Read the model definition and answer for the solid it produces. Units are mm, in the model's axes. Coordinates: 2 decimals unless noted, no trailing zeros. Order: outer loops, then holes, each group sorted by start corner. A loop starts at its lowest first (then second) coordinate and runs counter-clockwise, first axis right, second up. Notation, with made-up numbers: (28.5, -21) - (68.5, -21) arc R13 ccw to (68.5, -4) - close; hole circle Ø11 at (-3.75, 26.5). An arc over 180 degrees is marked (long way). Answer as a JSON object with one key per item and string values. Group by question number.
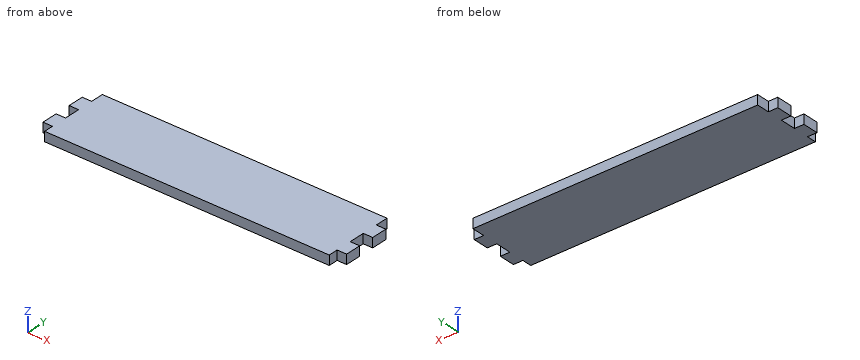
Autodesk Inventor part; units mm, degrees
ref_plane "YZ Plane" through (0, 0, 0) normal (1, 0, 0) x (0, 1, 0)
ref_plane "XZ Plane" through (0, 0, 0) normal (0, 1, 0) x (-1, 0, 0)
ref_plane "XY Plane" through (0, 0, 0) normal (0, 0, 1) x (1, 0, 0)
sketch "Эскиз1" plane through (0, 0, 0) normal (0, 0, 1) x (1, 0, 0)
  line L0 (0, 0) -> (0, -10)
  line L1 (0, 0) -> (-6, 0)
  line L2 (-6, -10) -> (-6, 0)
  line L3 (0, -10) -> (-6, -10)
  line L4 (0, -20) -> (0, -30)
  line L5 (0, -20) -> (-6, -20)
  line L6 (-6, -30) -> (-6, -20)
  line L7 (0, -30) -> (-6, -30)
  line L8 (0, -30) -> (0, -36.0265)
  line L9 (0, 8.1888) -> (0, 0)
  line L10 (186, -20) -> (186, -30)
  line L11 (186, -20) -> (180, -20)
  line L12 (180, -30) -> (180, -20)
  line L13 (186, -30) -> (180, -30)
  line L14 (186, 0) -> (186, -10)
  line L15 (186, 0) -> (180, 0)
  line L16 (180, -10) -> (180, 0)
  line L17 (186, -10) -> (180, -10)
  line L18 (180, -36.0265) -> (180, -30)
  line L19 (180, 0) -> (180, 8.1888)
  line L20 (0, 8.1888) -> (180, 8.1888)
  line L21 (180, 8.1888) -> (180, -36.0265)
  line L22 (180, -36.0265) -> (0, -36.0265)
  line L23 (0, -36.0265) -> (0, 8.1888)
extrude "Выдавливание1" add sketch "Эскиз1" along normal blind 6
properties part number "маленькое дно1"
1. Given pin 1 (3 mm diameter, centred on y = 6, z = 2.5, fed in from +X); pin 2 (1.8 mm diameter, centred on x = -4, z = 2, fed in from -Y); pin 3 (3 mm diameter, centred on x = 183.5, z = 2, fed in from +Y), each flat-ended and moving along its own axis, determine where each tip first touches the part or whether it passes through.
2. A cutting plane is placed at B-B on y = -16.5. Write down the section's boundary in (x, z), and give its area (3 significant figures).
3. A cutting plane is placed at A-A on z = 3.75. Write down the section's boundary in (x, y), and give its area (3 significant figures).
4. A straight line is drawn through the part: L1, parallel to X at y = -18, z = 3.2. Find the intervals that lie inside material, in ascending order.
Derived:
{
 "1": {"pin 1": "stops at x = 180", "pin 2": "stops at y = -30", "pin 3": "stops at y = 0"},
 "2": {"outline": "(0, 0) - (180, 0) - (180, 6) - (0, 6) - close", "area": "1,080 mm2"},
 "3": {"outline": "(-6, -30) - (0, -30) - (0, -36.03) - (180, -36.03) - (180, -30) - (186, -30) - (186, -20) - (180, -20) - (180, -10) - (186, -10) - (186, 0) - (180, 0) - (180, 8.19) - (0, 8.19) - (0, 0) - (-6, 0) - (-6, -10) - (0, -10) - (0, -20) - (-6, -20) - close", "area": "8,200 mm2"},
 "4": {"L1": "x = 0 to 180"}
}
